The model under review builds one solid part; all positions refer to its coordinate system, in mm. A direction names the side the tool comes from. Coordinates: 2 decimals unless noted, no trailing zeros. Write each loop counter-clockwise with the first axis right and the second up, starting at its lowest first coordinate (ties: lowest second). Pieces come first, ordered by that corner, then holes. Notation, with made-up numbers: M 20,28.5 L 37,28.5 A23 cw 37,42.5 Z; hole C -25,11 d4. An arc over 180 degrees is marked long. Answer as a JSON object with one key per item and string values.
Autodesk Inventor part; units mm, degrees
ref_plane "YZ Plane" through (0, 0, 0) normal (1, 0, 0) x (0, 1, 0)
ref_plane "XZ Plane" through (0, 0, 0) normal (0, 1, 0) x (-1, 0, 0)
ref_plane "XY Plane" through (0, 0, 0) normal (0, 0, 1) x (1, 0, 0)
sketch "Sketch1" plane through (0, 0, 0) normal (0, 1, 0) x (-1, 0, 0)
  line L0 (0, 0) -> (50, 0)
  line L1 (50, 0) -> (50, 20)
  line L2 (50, 20) -> (0, 20)
  line L3 (0, 20) -> (0, 0)
  dimension "d0" = 50
  dimension "d1" = 20
extrude "Extrusion1" add sketch "Sketch1" along normal blind 3
sketch "Sketch2" plane through (0, 3, 0) normal (0, 1, 0) x (1, 0, 0)
  line L0 (0, -20) -> (0, 0)
  line L1 (0, 0) -> (20, 0)
  line L2 (20, 0) -> (20, -20)
  line L3 (20, -20) -> (0, -20)
  line L4 (0, -20) -> (0, 0)
  dimension "d4" = 20
  dimension "d5" = 20
extrude "Extrusion2" add sketch "Sketch2" against normal blind 5
sketch "Sketch3" plane through (0, -2, 0) normal (0, -1, 0) x (1, 0, 0)
  point P0 (0, 0)
  point P1 (9.9251, 7.3531)
hole "Hole1" at (9.9251, -2, 7.3531) direction (0, 1, 0) diameter 7 end through all
properties part number "CameraTrainRig_holder_v2"
(1) For faces 4 (the face through (-25, 0, 10)), 5 (the face through (20, 1, 10)), list the 3-axis set-ups (+Z, -Z, +X, -X, +Y, -Y) from which the entire face can be reached by the end or side of a thin tool; tool diameter is ignored.
Results list:
{"face 4": "+Z, -Z, -X, -Y", "face 5": "+Z, -Z, +X, +Y, -Y"}
(2) For pin 1 Ø1.6 at (y, z) = (-1, 9) entering from -X; pin 2 Ø3 at (x, y) = (4, -0.5) entering from -Z; pin 3 Ø6 at (x, z) = (-21, 7) entering from -Y, all flat-tipped, find the tip position at first contact; note any pin that passes through.
Results list:
{"pin 1": "x = 0", "pin 2": "z = 0", "pin 3": "y = 0"}
(3) Add section B-B on z = 6.75. Give the boundary of the cut face in (x, y).
Results list:
{"outline": "M -50,0 L 0,0 L 0,-2 L 6.48,-2 L 6.48,3 L -50,3 Z; M 13.37,-2 L 20,-2 L 20,3 L 13.37,3 Z"}
(4) Draft analysis for pull direction X (two halves, no side actions). For faces 1 (the face through (-15, 3, 10)), 2 (the face through (0, -1, 10)), 3 (the face through (8.874, 0.535, 4.015)), state which applies: released by +X, released by -X, zero draft, split by the parting line, or undercut.
Results list:
{"face 1": "zero draft", "face 2": "released by -X", "face 3": "undercut"}
(5) Add section C-C on y = -1.15. Give the boundary of the cut face in (x, z).
Results list:
{"outline": "M 0,0 L 20,0 L 20,20 L 0,20 Z; hole C 9.93,7.35 d7"}
(6) Add section D-D on z = 18.75. Give the boundary of the cut face in (x, y), and give its area (3 significant figures).
Results list:
{"outline": "M -50,0 L 0,0 L 0,-2 L 20,-2 L 20,3 L -50,3 Z", "area": "250 mm²"}
(7) Add section A-A on x = 11.5. Give the boundary of the cut face in (y, z).
Results list:
{"outline": "M -2,0 L 3,0 L 3,4.23 L -2,4.23 Z; M -2,10.48 L 3,10.48 L 3,20 L -2,20 Z"}
(8) Wall thickness on line 1 along X through (y, z) = (1.35, 7.5); line 2 along Y through (x, z) = (-22.5, 1.5); line 3 along X through (y, z) = (-0.55, 7): over which ranges is each line inside the solid? List them lowest first. Write a range as from..to.
Results list:
{"line 1": "-50..6.43, 13.42..20", "line 2": "0..3", "line 3": "0..6.44, 13.41..20"}
